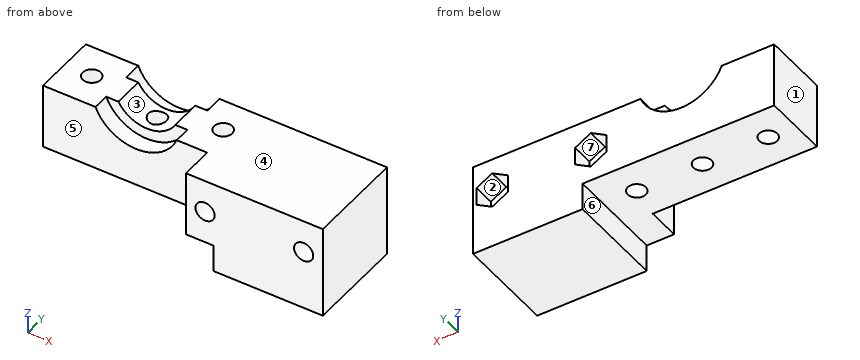
from build123d import *

# Parameters (mm, degrees)
EXTRUDE_1_DEPTH     = 3
EXTRUDE_2_DEPTH     = 5.6
EXTRUDE_3_DEPTH     = 3.4
SKETCH_5_W          = 25
SKETCH_5_H          = 12
EXTRUDE_4_DEPTH     = 18
SKETCH_8_W          = 20
SKETCH_8_H          = 18
EXTRUDE_5_DEPTH     = 5
SKETCH_4_R          = 1.65
CUT_EXTRUDE_1_DEPTH = 13
SKETCH_6_R          = 1.75
CUT_EXTRUDE_2_DEPTH = 19
CUT_EXTRUDE_3_DEPTH = 4


with BuildPart() as part:
    # 草图1 → 凸台-拉伸1 (new body)
    with BuildSketch(Plane(origin=(0, 0, 0), x_dir=(1, 0, 0), z_dir=(0, 1, 0))):
        with BuildLine():
            Line((17, 3), (17, 15))
            Line((17, 15), (-17, 15))
            Line((-17, 15), (-17, 3))
            Line((-17, 3), (-7.416198487, 3))
            ThreePointArc((-7.416198487, 3), (0, 8), (7.416198487, 3))
            Line((7.416198487, 3), (17, 3))
        make_face()
    extrude(amount=EXTRUDE_1_DEPTH)

    # 草图2 → 凸台-拉伸2 (add)
    with BuildSketch(Plane(origin=(0, 3, 0), x_dir=(1, 0, 0), z_dir=(0, 1, 0))):
        with BuildLine():
            Line((5.196152423, 3), (17, 3))
            Line((17, 3), (17, 15))
            Line((17, 15), (-17, 15))
            Line((-17, 15), (-17, 3))
            Line((-17, 3), (-5.196152423, 3))
            ThreePointArc((-5.196152423, 3), (0, 6), (5.196152423, 3))
        make_face()
    extrude(amount=EXTRUDE_2_DEPTH)

    # 草图3 → 凸台-拉伸3 (add)
    with BuildSketch(Plane(origin=(0, 8.6, 0), x_dir=(1, 0, 0), z_dir=(0, 1, 0))):
        with BuildLine():
            Line((-17, 3), (-7.416198487, 3))
            ThreePointArc((-7.416198487, 3), (0, 8), (7.416198487, 3))
            Line((7.416198487, 3), (17, 3))
            Line((17, 3), (17, 15))
            Line((17, 15), (-17, 15))
            Line((-17, 15), (-17, 3))
        make_face()
    extrude(amount=EXTRUDE_3_DEPTH)

    # 草图5 → 凸台-拉伸4 (add)
    with BuildSketch(Plane.XZ.offset(-12)):
        with Locations((25.5, -9)):
            Rectangle(SKETCH_5_W, SKETCH_5_H)
    extrude(amount=EXTRUDE_4_DEPTH)

    # 草图8 → 凸台-拉伸5 (add)
    with BuildSketch(Plane(origin=(0, 0, -15), x_dir=(-1, 0, 0), z_dir=(0, 0, -1))):
        with Locations((-28, 3)):
            Rectangle(SKETCH_8_W, SKETCH_8_H)
    extrude(amount=EXTRUDE_5_DEPTH)

    # 草图4 → 切除-拉伸1 (cut, through all)
    with BuildSketch(Plane.XY.offset(-15)):
        with Locations((-12, 6)):
            Circle(SKETCH_4_R)
        with Locations((12, 6)):
            Circle(SKETCH_4_R)
        with Locations((0, 6)):
            Circle(SKETCH_4_R)
    extrude(amount=CUT_EXTRUDE_1_DEPTH, mode=Mode.SUBTRACT)

    # 草图6 → 切除-拉伸2 (cut, through all)
    with BuildSketch(Plane.XZ.offset(6)):
        with Locations((16.5, -9)):
            Circle(SKETCH_6_R)
        with Locations((34.5, -9)):
            Circle(SKETCH_6_R)
    extrude(amount=-CUT_EXTRUDE_2_DEPTH, mode=Mode.SUBTRACT)

    # 草图7 → 切除-拉伸3 (cut)
    with BuildSketch(Plane(origin=(0, 12, 0), x_dir=(1, 0, 0), z_dir=(0, 1, 0))):
        Polygon((16.5, 5.709103466), (19.35, 7.354551733), (19.35, 10.645448267), (16.5, 12.290896534), (13.65, 10.645448267), (13.65, 7.354551733), align=None)
        Polygon((34.5, 5.709103466), (37.35, 7.354551733), (37.35, 10.645448267), (34.5, 12.290896534), (31.65, 10.645448267), (31.65, 7.354551733), align=None)
    extrude(amount=-CUT_EXTRUDE_3_DEPTH, mode=Mode.SUBTRACT)


solid = part.part
Geometry check sheet. Reference: the model listing, model coordinates, mm. Face numbers are marked on the shaded views. A direction names the side the tool comes from. Give positions to 0.01 mm unless a question says otherwise; leave off trailing zeros. Loops run counter-clockwise (first coordinate to the right, second up) from the corner with the lowest first, then second, coordinate; pieces in that order, holes last. Notation, with made-up numbers: M -21.5,87.5 L 25.5,87.5 A23 cw 25.5,121.5 Z; hole C -16,46.5 d2. An arc over 180 degrees is marked long. Answer as a JSON object with one key per item and string values. Group by question number.
Item 1: Access from +Z, -Z, +X, -X, +Y, -Y to the whole of each face (thin tool, end or side, straight path). Record for the marked faces 5, 6 and 7.
Item 2: Material ranges on L1, parallel to X at y = 6, z = -6.5; L2, parallel to Y at x = 12, z = -11; L3, parallel to Z at x = 16.5, y = 0.25, recorded low to high.
Item 3: Sectioned sample at B-B on x = -12. Record the boundary of the cut face in (y, z).
Item 4: Mould release check, pull along X, two halves, no side actions. Record for the marked faces 1, 2, 3 and 4: pulls with the +X half, pulls with the -X half, needs draft (parallel to the pull), parting line crosses it, or undercut.
Item 5: Sectioned sample at C-C on y = 2.5. Record the boundary of the cut face in (x, z).
Item 6: Sectioned sample at A-A on y = 6. Record the boundary of the cut face in (x, z).
Item 7: Gauge pin test, flat ends, axial feed: pin 1 (4 mm diameter, centred on y = 6.5, z = -18.5, fed in from -X); pin 2 (4 mm diameter, centred on x = 0.5, z = -4.5, fed in from -Y); pin 3 (1.7 mm diameter, centred on x = 33.5, z = -10.5, fed in from +Y). Record the tip position at first contact, or that the pin passes through.
Item 8: Sectioned sample at D-D on x = 0. Record the boundary of the cut face in (y, z).
Findings below:
{
 "1": {"face 5": "+Z, -Z, -X, -Y", "face 6": "-Z, -X, +Y, -Y", "face 7": "+Y"},
 "2": {"L1": "-17 to -13.65, -10.35 to -1.65, 1.65 to 10.35, 13.65 to 38", "L2": "0 to 4.35, 7.65 to 12", "L3": "-15 to -10.75, -7.25 to -3"},
 "3": {"outline": "M 0,-15 L 4.35,-15 L 4.35,-3 L 0,-3 Z; M 7.65,-15 L 12,-15 L 12,-3 L 7.65,-3 Z"},
 "4": {"face 1": "pulls with the -X half", "face 2": "undercut", "face 3": "undercut", "face 4": "needs draft"},
 "5": {"outline": "M -17,-15 L 18,-15 L 18,-20 L 38,-20 L 38,-3 L 7.42,-3 A8 cw -7.42,-3 L -17,-3 Z; hole C 16.5,-9 d3.5; hole C 34.5,-9 d3.5"},
 "6": {"outline": "M -17,-15 L -13.65,-15 L -13.65,-3 L -17,-3 Z; M -10.35,-15 L -1.65,-15 L -1.65,-5.77 A6 cw -5.2,-3 L -10.35,-3 Z; M 1.65,-15 L 10.35,-15 L 10.35,-3 L 5.2,-3 A6 cw 1.65,-5.77 Z; M 13.65,-15 L 18,-15 L 18,-20 L 38,-20 L 38,-3 L 13.65,-3 Z; hole C 16.5,-9 d3.5; hole C 34.5,-9 d3.5"},
 "7": {"pin 1": "x = 18", "pin 2": "y = 3", "pin 3": "y = 8"},
 "8": {"outline": "M 0,-15 L 4.35,-15 L 4.35,-6 L 3,-6 L 3,-8 L 0,-8 Z; M 7.65,-15 L 12,-15 L 12,-8 L 8.6,-8 L 8.6,-6 L 7.65,-6 Z"}
}
